```python
from build123d import *

# Parameters (mm, degrees)
SKETCH_R      = 1.575
SKETCH_R_2    = 1.6
PAD_DEPTH     = 3
SKETCH001_R   = 3.5
SKETCH001_R_2 = 1.575
PAD001_DEPTH  = 7


with BuildPart() as part:
    # Sketch → Pad (new body)
    with BuildSketch(Plane.XY):
        with BuildLine():
            Line((-10, 8.5), (10, 8.5))
            Line((10, 8.5), (10, -1.5))
            Line((10, -1.5), (19.3418018487, -2.4167297699))
            ThreePointArc((18.6581766844, -9.3832681236), (22.4832691769, -6.2418125822), (19.3418018487, -2.4167297699))
            Line((18.6581766844, -9.3832681236), (3.5183762437, -7.897569112))
            Line((3.5183762437, -7.897569112), (3.5183762437, -46.5971976167))
            Line((3.5183762437, -46.5971976167), (17.867093033, -41.6884260835))
            ThreePointArc((20.1329069981, -48.3115739058), (22.3115739111, -43.8670930175), (17.867093033, -41.6884260835))
            Line((1.1329067211, -54.8115740006), (20.1329069981, -48.3115739058))
            ThreePointArc((-1.1409673211, -54.80880546), (-0.0042613991, -54.9999974058), (1.1329067211, -54.8115740006))
            Line((-19.9909670183, -48.3088055644), (-1.1409673211, -54.80880546))
            ThreePointArc((-17.7090326253, -41.6911945585), (-22.158805503, -43.8590328035), (-19.9909670183, -48.3088055644))
            Line((-3.4816237563, -46.5971976167), (-17.7090326253, -41.6911945585))
            Line((-3.4816237563, -7.8846304044), (-3.4816237563, -46.5971976167))
            Line((-3.4816237563, -7.8846304044), (-18.5026576912, -9.3827221136))
            ThreePointArc((-19.1973406361, -2.4172777196), (-22.332722197, -6.2473414725), (-18.5026576912, -9.3827221136))
            Line((-10, -1.5), (-19.1973406361, -2.4172777196))
            Line((-10, 8.5), (-10, -1.5))
        make_face()
        with Locations((-18.85, -45)):
            Circle(SKETCH_R, mode=Mode.SUBTRACT)
        with Locations((19, -45)):
            Circle(SKETCH_R, mode=Mode.SUBTRACT)
        with Locations((0, -51.5)):
            Circle(SKETCH_R_2, mode=Mode.SUBTRACT)
        with Locations((0, 3.5)):
            Circle(SKETCH_R_2, mode=Mode.SUBTRACT)
        with Locations((-18.85, -5.9)):
            Circle(SKETCH_R, mode=Mode.SUBTRACT)
        with Locations((19, -5.9)):
            Circle(SKETCH_R, mode=Mode.SUBTRACT)
    extrude(amount=PAD_DEPTH)

    # Sketch001 → Pad001 (new body)
    with BuildSketch(Plane.XY.offset(3)):
        with Locations((-18.85, -5.9)):
            Circle(SKETCH001_R)
        with Locations((-18.85, -5.9)):
            Circle(SKETCH001_R_2, mode=Mode.SUBTRACT)
        with Locations((19, -5.9)):
            Circle(SKETCH001_R)
        with Locations((19, -5.9)):
            Circle(SKETCH001_R_2, mode=Mode.SUBTRACT)
        with Locations((19, -45)):
            Circle(SKETCH001_R)
        with Locations((19, -45)):
            Circle(SKETCH001_R_2, mode=Mode.SUBTRACT)
        with Locations((-18.85, -45)):
            Circle(SKETCH001_R)
        with Locations((-18.85, -45)):
            Circle(SKETCH001_R_2, mode=Mode.SUBTRACT)
    extrude(amount=PAD001_DEPTH)


solid = part.part
```
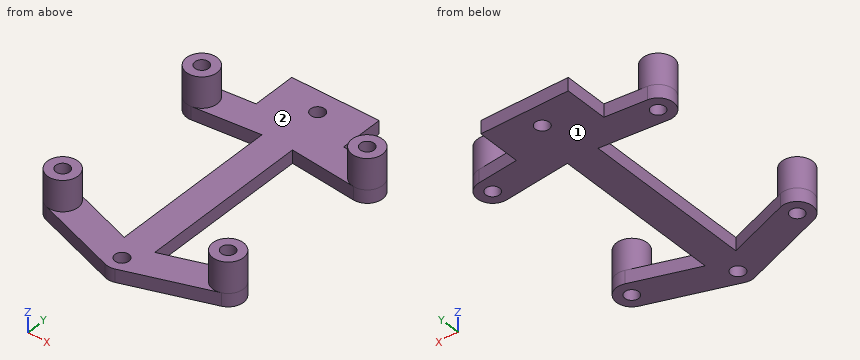
Can you work these out from the model? Positions are in its coordinate system, mm. Face numbers are marked on the shaded views. Give positions to 0.01 mm unless a question says otherwise; leave off trailing zeros. Order: outer loops, then holes, each group sorted by start corner. A loop starts at its lowest first (then second) coordinate and runs counter-clockwise, first axis right, second up. Notation, with made-up numbers: M -25.75,32.5 L 19.25,32.5 A20 ccw 19.25,37.5 Z; hole C 55.5,70 d10. An arc over 180 degrees is marked long. Write item = value, one per line. Start each with the question number.
Q1. Suppose I cut it at A-A (z = 7.5). Write out the boundary of the cut face in (x, y) (3 decimals), plus the area to 3 significant figures.
Q2. Suppose I cut it at D-D (y = -5.9). Write out the boundary of the cut face in (x, z) (3 decimals), plus the area to 3 significant figures.
Q3. I need wall thicknesses on probe 1 along Y at (x, z) = (-18.85, 3.75) (3 decimals); probe 2 along Y at (x, z) = (0, 1.8); probe 3 along Z at (x, y) = (5, -48). Which ranges of each line are inside material? Lowest first, please. Write a range as [from, to].
Q4. Suppose I cut it at C-C (x = 0). Write out the boundary of the cut face in (y, z), plus the area to 3 significant figures.
Q5. Suppose I cut it at B-B (y = 3.5). Write out the boundary of the cut face in (x, z).
Q6. We'd pull the mould along X, two halves only. Please class the marked faces 1 and 2: pulls with the +X half, pulls with the -X half, needs draft (parallel to the pull), parting line crosses it, or undercut.
Q7. Will these pins go through, and if not, where does the flat tip stop? pin 1 Ø0.9 at (y, z) = (-26.5, 1.5) entering from -X; pin 2 Ø0.9 at (y, z) = (4, 1) entering from -X; pin 3 Ø12 at (x, y) = (5.5, -10.5) entering from +Z.
Check result:
q1.outline = C -18.85,-45 d7; C -18.85,-5.9 d7; C 19,-45 d7; C 19,-5.9 d7; hole C -18.85,-45 d3.15; hole C -18.85,-5.9 d3.15; hole C 19,-45 d3.15; hole C 19,-5.9 d3.15
q1.area = 123 mm2
q2.outline = M -22.35,0 L -20.425,0 L -20.425,10 L -22.35,10 Z; M -17.275,0 L 17.425,0 L 17.425,10 L 15.5,10 L 15.5,3 L -15.35,3 L -15.35,10 L -17.275,10 Z; M 20.575,0 L 22.5,0 L 22.5,10 L 20.575,10 Z
q2.area = 170 mm2
q3.probe_1 = [-48.5, -46.575], [-43.425, -41.5], [-9.4, -7.475], [-4.325, -2.4]
q3.probe_2 = [-55, -53.1], [-49.9, 1.9], [5.1, 8.5]
q3.probe_3 = [0, 3]
q4.outline = M -55,0 L -53.1,0 L -53.1,3 L -55,3 Z; M -49.9,0 L 1.9,0 L 1.9,3 L -49.9,3 Z; M 5.1,0 L 8.5,0 L 8.5,3 L 5.1,3 Z
q4.area = 171 mm2
q5.outline = M -10,0 L -1.6,0 L -1.6,3 L -10,3 Z; M 1.6,0 L 10,0 L 10,3 L 1.6,3 Z
q6.face_1 = needs draft
q6.face_2 = undercut
q7.pin_1 = -3.48
q7.pin_2 = -10
q7.pin_3 = 3
